The model under review builds one solid part; all positions refer to its coordinate system, in mm. Face numbers are marked on the shaded views. Round coordinates to 2 decimals unless told otherwise and drop trailing zeros. Order: outer loops, then holes, each group sorted by start corner. A loop starts at its lowest first (then second) coordinate and runs counter-clockwise, first axis right, second up. Notation, with made-up numbers: M 1.25,-1 L 40.25,-1 A12 cw 40.25,10 Z; hole C 21.5,59 d7. An arc over 180 degrees is marked long. One line per item, written item: value. Start each with the question number.
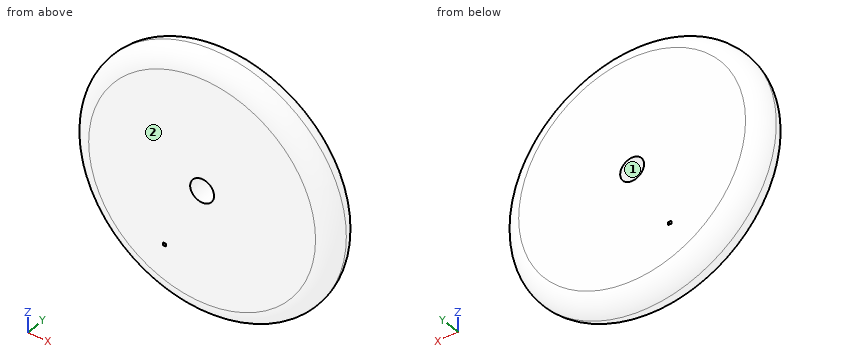
from build123d import *

# Parameters (mm, degrees)
F0_R     = 6.985
F0_W     = 0.1642033458
F0_H     = 0.1596324146
F0_R_2   = 0.635
F1_DEPTH = 1.905
F2_R     = 0.95249


# Not quite as in the source:
# - a fillet or chamfer is up to 0.001 mm smaller than in the source, because OpenCascade refuses the exact size


with BuildPart() as f1:
    # F0 (on Front) → F1 (new body)
    with BuildSketch(Plane.XZ):
        with Locations((-56.4259625971, 38.3895114064)):
            Circle(F0_R)
        with Locations((-58.4293603897, 34.6161220223)):
            Rectangle(F0_W, F0_H, mode=Mode.SUBTRACT)
        with Locations((-56.4259625971, 38.3895114064)):
            Circle(F0_R_2, mode=Mode.SUBTRACT)
    extrude(amount=F1_DEPTH)

    # F2 (radius 0.9525 in the source; OpenCascade refuses exactly that, so slightly less here)
    f2_edges = [f1.edges().sort_by_distance(p)[0] for p in [
        (-63.410963, -1.905, 38.389511),
        (-63.410963, 0, 38.389511),
    ]]
    fillet(f2_edges, radius=F2_R)


solid = f1.part
Item 1: Clearance check with a flat-ended pin moving along its axis: P1, Ø1, axis at y = 0, z = 40.5, coming from the +X side. State where the tip first meets the part, or that it passes through.
Item 2: The part is to be moulded in two halves that separate along X. For the marked faces 1 and 2, say which applies: pulls with the +X half, pulls with the -X half, needs draft (parallel to the pull), parting line crosses it, or undercut.
Item 3: Consider section B-B, the plane y = -1.2. Give the boundary of the cut face in (x, z) (3 decimals).
Item 4: Consider section A-A, the plane y = -0.3. Give the boundary of the cut face in (x, z) (3 decimals), then the cut area to 3 significant figures.
Item 5: Wall thickness on L1, parallel to Y at x = -51.75, z = 34.5; L2, parallel to Z at x = -62, y = -0.5; L3, parallel to Z at x = -50.25, y = -0.9: over which ranges is each line inside the solid? List them lowest first.
Computed:
1. P1: stops at x = -49.85
2. face 1: undercut
2. face 2: needs draft
3. outline: C -56.426,38.39 d13.905; hole M -58.511,34.536 L -58.347,34.536 L -58.347,34.696 L -58.511,34.696 Z; hole C -56.426,38.39 d1.27
4. outline: C -56.426,38.39 d13.453; hole M -58.511,34.536 L -58.347,34.536 L -58.347,34.696 L -58.511,34.696 Z; hole C -56.426,38.39 d1.27
4. area: 141 mm^2
5. L1: y = -1.9 to 0
5. L2: z = 34.37 to 42.41
5. L3: z = 35.13 to 41.65
